```python
from build123d import *

# Parameters (mm, degrees)
SKETCH_1_W          = 36
SKETCH_1_H          = 21
SKETCH_1_R          = 1.25
SKETCH_1_R_2        = 1.3
SKETCH_1_R_3        = 1.35
EXTRUDE_1_DEPTH     = 140
SKETCH_1_5_R        = 1.3
SKETCH_1_5_R_2      = 1.35
SKETCH_1_5_R_3      = 1.25
CUT_EXTRUDE_1_DEPTH = 4
CUT_EXTRUDE_START   = 140
SKETCH_1_6_R        = 1.35
SKETCH_1_6_R_2      = 1.3
SKETCH_1_6_R_3      = 1.25
CUT_EXTRUDE_2_DEPTH = 4
CUT_EXTRUDE_3_REACH = 144.706
FILLET_1_R          = 1.5


with BuildPart() as part:
    # 스케치1 → 보스-돌출1 (new body)
    with BuildSketch(Plane.XY):
        Rectangle(SKETCH_1_W, SKETCH_1_H)
        with Locations((-3.5, -8)):
            Circle(SKETCH_1_R, mode=Mode.SUBTRACT)
        with Locations((3.5, -8)):
            Circle(SKETCH_1_R, mode=Mode.SUBTRACT)
        with Locations((-12, 6)):
            Circle(SKETCH_1_R_2, mode=Mode.SUBTRACT)
        with Locations((12, 6)):
            Circle(SKETCH_1_R_2, mode=Mode.SUBTRACT)
        with Locations((12, -6)):
            Circle(SKETCH_1_R_2, mode=Mode.SUBTRACT)
        with Locations((-12, -6)):
            Circle(SKETCH_1_R_2, mode=Mode.SUBTRACT)
        with Locations((3.5, 8)):
            Circle(SKETCH_1_R_3, mode=Mode.SUBTRACT)
        with Locations((-3.5, 8)):
            Circle(SKETCH_1_R_3, mode=Mode.SUBTRACT)
        with Locations((12, -6)):
            Circle(SKETCH_1_R_2)
        with Locations((3.5, -8)):
            Circle(SKETCH_1_R)
        with Locations((-3.5, -8)):
            Circle(SKETCH_1_R)
        with Locations((-12, -6)):
            Circle(SKETCH_1_R_2)
        with Locations((-12, 6)):
            Circle(SKETCH_1_R_2)
        with Locations((-3.5, 8)):
            Circle(SKETCH_1_R_3)
        with Locations((3.5, 8)):
            Circle(SKETCH_1_R_3)
        with Locations((12, 6)):
            Circle(SKETCH_1_R_2)
    extrude(amount=EXTRUDE_1_DEPTH)

    # 스케치1<5> → 컷-돌출1 (cut)
    with BuildSketch(Plane.XY):
        with Locations((12, 6)):
            Circle(SKETCH_1_5_R)
        with Locations((3.5, 8)):
            Circle(SKETCH_1_5_R_2)
        with Locations((-3.5, 8)):
            Circle(SKETCH_1_5_R_2)
        with Locations((-12, 6)):
            Circle(SKETCH_1_5_R)
        with Locations((-12, -6)):
            Circle(SKETCH_1_5_R)
        with Locations(Location((-3.5, -8, 0), (0, 0, 180))):
            Circle(SKETCH_1_5_R_3)
        with Locations((3.5, -8)):
            Circle(SKETCH_1_5_R_3)
        with Locations((12, -6)):
            Circle(SKETCH_1_5_R)
    extrude(amount=CUT_EXTRUDE_1_DEPTH, mode=Mode.SUBTRACT)

    # 스케치1<6> → 컷-돌출2 (cut)
    with BuildSketch(Plane.XY.offset(CUT_EXTRUDE_START)):
        with Locations((3.5, 8)):
            Circle(SKETCH_1_6_R)
        with Locations((12, 6)):
            Circle(SKETCH_1_6_R_2)
        with Locations((-3.5, 8)):
            Circle(SKETCH_1_6_R)
        with Locations((-12, 6)):
            Circle(SKETCH_1_6_R_2)
        with Locations((-12, -6)):
            Circle(SKETCH_1_6_R_2)
        with Locations(Location((-3.5, -8, 0), (0, 0, 180))):
            Circle(SKETCH_1_6_R_3)
        with Locations((3.5, -8)):
            Circle(SKETCH_1_6_R_3)
        with Locations((12, -6)):
            Circle(SKETCH_1_6_R_2)
    extrude(amount=-CUT_EXTRUDE_2_DEPTH, mode=Mode.SUBTRACT)

    # 스케치2 → 컷-돌출3 (cut, up to next)
    with BuildSketch(Plane(origin=(0, 10.5, 0), x_dir=(1, 0, 0), z_dir=(0, 1, 0)), mode=Mode.PRIVATE) as cut_extrude_3_sk1:
        with BuildLine():
            Line((7.5, -15), (7.5, -57))
            ThreePointArc((7.5, -57), (0, -64.5), (-7.5, -57))
            Line((-7.5, -57), (-7.5, -15))
            ThreePointArc((-7.5, -15), (0, -7.5), (7.5, -15))
        make_face()
    cut_extrude_3_tool1 = extrude(cut_extrude_3_sk1.sketch, amount=-CUT_EXTRUDE_3_REACH, mode=Mode.PRIVATE) & part.part
    # 스케치2 → 컷-돌출3 (cut, up to next)
    with BuildSketch(Plane(origin=(0, 10.5, 0), x_dir=(1, 0, 0), z_dir=(0, 1, 0)), mode=Mode.PRIVATE) as cut_extrude_3_sk2:
        with BuildLine():
            Line((7.5, -125), (7.5, -83))
            ThreePointArc((7.5, -83), (0, -75.5), (-7.5, -83))
            Line((-7.5, -83), (-7.5, -125))
            ThreePointArc((-7.5, -125), (0, -132.5), (7.5, -125))
        make_face()
    cut_extrude_3_tool2 = extrude(cut_extrude_3_sk2.sketch, amount=-CUT_EXTRUDE_3_REACH, mode=Mode.PRIVATE) & part.part
    add(cut_extrude_3_tool1.solids().sort_by_distance((0, 10.5, 36))[0], mode=Mode.SUBTRACT)
    add(cut_extrude_3_tool2.solids().sort_by_distance((0, 10.5, 104))[0], mode=Mode.SUBTRACT)

    # 필렛1
    fillet_1_edges = [part.edges().sort_by_distance(p)[0] for p in [
        (0, -10.5, 7.5),
        (7.5, -10.5, 36),
        (0, -10.5, 64.5),
        (-7.5, -10.5, 36),
        (0, 10.5, 7.5),
        (-18, 10.5, 70),
        (-7.5, 10.5, 36),
        (0, 10.5, 64.5),
        (7.5, 10.5, 36),
        (18, 10.5, 70),
        (18, -10.5, 70),
        (-18, -10.5, 70),
        (0, -10.5, 132.5),
        (-7.5, -10.5, 104),
        (0, -10.5, 75.5),
        (7.5, -10.5, 104),
        (0, 10.5, 132.5),
        (7.5, 10.5, 104),
        (0, 10.5, 75.5),
        (-7.5, 10.5, 104),
    ]]
    fillet(fillet_1_edges, radius=FILLET_1_R)


solid = part.part
```
CAD build for the part. Positions are in the model's coordinates, mm. A direction names the side the tool comes from. Round coordinates to 2 decimals unless told otherwise and drop trailing zeros. Order: outer loops, then holes, each group sorted by start corner. A loop starts at its lowest first (then second) coordinate and runs counter-clockwise, first axis right, second up.
Item 1: Saw through at A-A on y = 2. Write the cut outline in (x, z), then the cut area to 3 significant figures.
Item 2: Probe line 1 along Y through (x, z) = (-3.5, 138.2); line 2 along Y through (x, z) = (-12, 2.45); line 3 along Z through (x, y) = (0.5, 5). List the from-to ranges inside material, lowest first.
Item 3: Mould opens along Y. For faces 6 (the face through (7.5, 0, 104)), 7 (the face through (0, -10.5, 69)), 8 (the face through (-12, 6, 4)) say: pulls with the +Y half, pulls with the -Y half, needs draft (parallel to the pull), parting line crosses it, or undercut.
Item 4: Pin check, flat tips, straight feed: pin 1 (0.8 mm diameter, centred on x = -3, y = 8.5, fed in from -Z); pin 2 (1.3 mm diameter, centred on x = -12.5, y = -6, fed in from +Z); pin 3 (2 mm diameter, centred on x = -7.5, z = 124.5, fed in from -Y); pin 4 (10 mm diameter, centred on x = -0.5, z = 54, fed in from -Y). Stop position of each tip, or through.
Item 5: Tool access for faces 1 (the face through (-18, 0, 69)), 2 (the face through (12.6, -7.153, 1.972)), 3 (the face through (-7.5, 0, 36)), 4 (the face through (12, -6, 136)), 5 (the face through (0, 0, 140)): list every direction of +Z, -Z, +X, -X, +Y, -Y with a clear straight run to the whole face (end or side of a thin tool).
Reported:
1. outline: (-18, 0) - (18, 0) - (18, 140) - (-18, 140) - close; hole (-7.5, 15) arc R7.5 ccw to (7.5, 15) - (7.5, 57) arc R7.5 ccw to (-7.5, 57) - close; hole (-7.5, 83) arc R7.5 ccw to (7.5, 83) - (7.5, 125) arc R7.5 ccw to (-7.5, 125) - close
1. area: 3,430 mm2
2. line 1: y = -10.5 to -9.25, -6.75 to 6.65, 9.35 to 10.5
2. line 2: y = -10.5 to -7.3, -4.7 to 4.7, 7.3 to 10.5
2. line 3: z = 0 to 7.52, 64.48 to 75.52, 132.48 to 140
3. face 6: needs draft
3. face 7: pulls with the -Y half
3. face 8: undercut
4. pin 1: stops at z = 4
4. pin 2: stops at z = 136
4. pin 3: stops at y = -10.41
4. pin 4: passes through
5. face 1: +Z, -Z, -X, +Y, -Y
5. face 2: -Z
5. face 3: +Y, -Y
5. face 4: +Z
5. face 5: +Z, +X, -X, +Y, -Y
